Geometry: final body of the model. Coordinates: model frame, mm. A direction names the side the tool comes from. Give positions to 0.01 mm unless a question says otherwise; leave off trailing zeros. Write each loop counter-clockwise with the first axis right and the second up, starting at its lowest first coordinate (ties: lowest second). Pieces come first, ordered by that corner, then holes. Notation, with made-up numbers: (79.25, -10) -> (109.25, -10) arc R11 cw to (109.25, 3) -> close; hole circle Ø6 at (35, 68.25). An arc over 180 degrees is marked (long way). Use CSV: the item, a comma, the result in double quotes. Start each with the question number.
1) Material intervals for line 1 (Y direction, x = 249, z = 56); line 2 (Y direction, x = 108, z = 0), sorted ascending. Write a range as [from, to].
2) Contact query for flat-ended pins moving along their axis: P1, Ø6, axis at x = 129.5, y = -0.5, coming from the +Z side; P2, Ø1, axis at x = 158, y = 28, coming from the +Z side; P3, Ø24.5, axis at y = 97.86, z = -56.5, coming from the -X side. Output: stop coordinate, or through.
3) Section A-A (z = 99.5). Output: boundary loops of the cut face in (x, y), plus the area to 3 significant figures.
4) Draft query along X for faces 4 (the face through (13.846, 15.703, 37.874)), 5 (the face through (0, -10.6, 29.4)), 6 (the face through (1.479, 39.923, 20.765)). Return one class per face: pulls with the +X half, pulls with the -X half, needs draft (parallel to the pull), parting line crosses it, or undercut.
5) Section D-D (x = 57). Output: boundary loops of the cut face in (y, z), plus the area to 3 significant figures.
6) Section B-B (z = -113). Output: boundary loops of the cut face in (x, y), plus the area to 3 significant figures.
7) Set-up query: faces 1 (the face through (145.063, -15.77, 50.076)), 2 (the face through (106.482, -19.674, 62.475)), 3 (the face through (251.818, 59.354, -106.922)). Return all of +Z, -Z, +X, -X, +Y, -Y with unobstructed straight access to the full face (end or side cutting, diameter ignored); none if empty.
```python
from build123d import *

# Parameters (mm, degrees)
SKETCH_3_R           = 9.5
CUT_EXTRUDE_1_DEPTH  = 321.526909947
SKETCH_4_R           = 9.5
CUT_EXTRUDE_2_DEPTH  = 321.526909947
SKETCH_5_R           = 9.5
CUT_EXTRUDE_3_DEPTH  = 321.526909947
SKETCH_6_R           = 9.5
CUT_EXTRUDE_4_DEPTH  = 321.526909947
SKETCH_7_R           = 9.5
CUT_EXTRUDE_5_DEPTH  = 321.526909947
SKETCH_8_R           = 9.5
CUT_EXTRUDE_6_DEPTH  = 321.526909947
SKETCH_9_R           = 9.5
CUT_EXTRUDE_7_DEPTH  = 321.526909947
SKETCH_10_R          = 9.5
CUT_EXTRUDE_8_DEPTH  = 321.526909947
SKETCH_11_R          = 9.5
CUT_EXTRUDE_9_DEPTH  = 321.526909947
SKETCH_12_R          = 9.5
CUT_EXTRUDE_10_DEPTH = 321.526909947
SKETCH_13_R          = 9.5
CUT_EXTRUDE_11_DEPTH = 321.526909947
SKETCH_14_R          = 9.5
CUT_EXTRUDE_12_DEPTH = 321.526909947


with BuildPart() as part:
    # Эскиз1 → Повернуть1 (revolve)
    with BuildSketch(Plane.XY, mode=Mode.PRIVATE) as revolve_1_sk:
        Polygon((0, 0), (265, 0), (265, 127.5), (239, 127.5), (239, 100), (239, 95), (220, 95), (220, 94), (200, 94), (144, 65.5), (70, 65.5), (25, 41), (3, 41), (3, 45), (0, 45), align=None)
    revolve(revolve_1_sk.sketch.rotate(Axis((0, 0, 0), (1, 0, 0)), 90), axis=Axis((0, 0, 0), (1, 0, 0)))

    # Эскиз2 → Вырез-Повернуть1 (revolve, cut)
    with BuildSketch(Plane.XY, mode=Mode.PRIVATE) as cut_revolve_1_sk:
        with BuildLine():
            Line((0, 0), (239, 0))
            Line((239, 0), (239, 47))
            Line((239, 47), (210, 47))
            ThreePointArc((210, 47), (209, 47.16088641), (208, 47))
            Line((208, 47), (200, 55))
            Line((200, 55), (147.669872, 55))
            ThreePointArc((147.669872, 55), (146.273624348, 54.108499061), (146.669872, 52.5))
            Line((146.669872, 52.5), (143.5, 52.5))
            ThreePointArc((143.5, 52.5), (142.75, 52.602347572), (142, 52.5))
            Line((142, 52.5), (90, 52.5))
            ThreePointArc((90, 52.5), (79.13262933, 46.740617582), (70, 38.502577))
            Line((70, 38.502577), (42, 31))
            Line((42, 31), (0, 31))
            Line((0, 31), (0, 0))
        make_face()
    revolve(cut_revolve_1_sk.sketch.rotate(Axis((0, 0, 0), (1, 0, 0)), 90), axis=Axis((0, 0, 0), (1, 0, 0)), mode=Mode.SUBTRACT)

    # Эскиз3 → Вырез-Вытянуть1 (cut, through all)
    with BuildSketch(Plane(origin=(0, 0, 0), x_dir=(0, 0, -1), z_dir=(1, 0, 0))):
        with Locations((0, 113)):
            Circle(SKETCH_3_R)
    extrude(amount=CUT_EXTRUDE_1_DEPTH, mode=Mode.SUBTRACT)

    # Эскиз4 → Вырез-Вытянуть2 (cut, through all)
    with BuildSketch(Plane(origin=(0, 0, 0), x_dir=(0, 0, -1), z_dir=(1, 0, 0))):
        with Locations((-56.5, 97.860870628)):
            Circle(SKETCH_4_R)
    extrude(amount=CUT_EXTRUDE_2_DEPTH, mode=Mode.SUBTRACT)

    # Эскиз5 → Вырез-Вытянуть3 (cut, through all)
    with BuildSketch(Plane(origin=(0, 0, 0), x_dir=(0, 0, -1), z_dir=(1, 0, 0))):
        with Locations((-97.860870628, 56.5)):
            Circle(SKETCH_5_R)
    extrude(amount=CUT_EXTRUDE_3_DEPTH, mode=Mode.SUBTRACT)

    # Эскиз6 → Вырез-Вытянуть4 (cut, through all)
    with BuildSketch(Plane(origin=(0, 0, 0), x_dir=(0, 0, -1), z_dir=(1, 0, 0))):
        with Locations((-113, 0)):
            Circle(SKETCH_6_R)
    extrude(amount=CUT_EXTRUDE_4_DEPTH, mode=Mode.SUBTRACT)

    # Эскиз7 → Вырез-Вытянуть5 (cut, through all)
    with BuildSketch(Plane(origin=(0, 0, 0), x_dir=(0, 0, -1), z_dir=(1, 0, 0))):
        with Locations((-97.860870628, -56.5)):
            Circle(SKETCH_7_R)
    extrude(amount=CUT_EXTRUDE_5_DEPTH, mode=Mode.SUBTRACT)

    # Эскиз8 → Вырез-Вытянуть6 (cut, through all)
    with BuildSketch(Plane(origin=(0, 0, 0), x_dir=(0, 0, -1), z_dir=(1, 0, 0))):
        with Locations((-56.5, -97.860870628)):
            Circle(SKETCH_8_R)
    extrude(amount=CUT_EXTRUDE_6_DEPTH, mode=Mode.SUBTRACT)

    # Эскиз9 → Вырез-Вытянуть7 (cut, through all)
    with BuildSketch(Plane(origin=(0, 0, 0), x_dir=(0, 0, -1), z_dir=(1, 0, 0))):
        with Locations((0, -113)):
            Circle(SKETCH_9_R)
    extrude(amount=CUT_EXTRUDE_7_DEPTH, mode=Mode.SUBTRACT)

    # Эскиз10 → Вырез-Вытянуть8 (cut, through all)
    with BuildSketch(Plane(origin=(0, 0, 0), x_dir=(0, 0, -1), z_dir=(1, 0, 0))):
        with Locations((56.5, -97.860870628)):
            Circle(SKETCH_10_R)
    extrude(amount=CUT_EXTRUDE_8_DEPTH, mode=Mode.SUBTRACT)

    # Эскиз11 → Вырез-Вытянуть9 (cut, through all)
    with BuildSketch(Plane(origin=(0, 0, 0), x_dir=(0, 0, -1), z_dir=(1, 0, 0))):
        with Locations((97.860870628, -56.5)):
            Circle(SKETCH_11_R)
    extrude(amount=CUT_EXTRUDE_9_DEPTH, mode=Mode.SUBTRACT)

    # Эскиз12 → Вырез-Вытянуть10 (cut, through all)
    with BuildSketch(Plane(origin=(0, 0, 0), x_dir=(0, 0, -1), z_dir=(1, 0, 0))):
        with Locations((113, 0)):
            Circle(SKETCH_12_R)
    extrude(amount=CUT_EXTRUDE_10_DEPTH, mode=Mode.SUBTRACT)

    # Эскиз13 → Вырез-Вытянуть11 (cut, through all)
    with BuildSketch(Plane(origin=(0, 0, 0), x_dir=(0, 0, -1), z_dir=(1, 0, 0))):
        with Locations((97.860870628, 56.5)):
            Circle(SKETCH_13_R)
    extrude(amount=CUT_EXTRUDE_11_DEPTH, mode=Mode.SUBTRACT)

    # Эскиз14 → Вырез-Вытянуть12 (cut, through all)
    with BuildSketch(Plane(origin=(0, 0, 0), x_dir=(0, 0, -1), z_dir=(1, 0, 0))):
        with Locations((56.5, 97.860870628)):
            Circle(SKETCH_14_R)
    extrude(amount=CUT_EXTRUDE_12_DEPTH, mode=Mode.SUBTRACT)


solid = part.part
```
Answers follow:
1,line 1,"y = [-114.54, -107.35], [-88.37, 88.37], [107.35, 114.54]"
1,line 2,"y = [-65.5, -52.5], [52.5, 65.5]"
2,P1,"stops at z = 65.5"
2,P2,"stops at z = 67.36"
2,P3,"stops at x = 239"
3,outline,"(239, -79.72) -> (265, -79.72) -> (265, -65.86) -> (239, -65.86) -> close; (239, -47.14) -> (265, -47.14) -> (265, 47.14) -> (239, 47.14) -> close; (239, 65.86) -> (265, 65.86) -> (265, 79.72) -> (239, 79.72) -> close"
3,area,"3,170 mm^2"
4,face 4,"undercut"
4,face 5,"pulls with the -X half"
4,face 6,"needs draft"
5,outline,"circle Ø116.84 at (0, 0); hole circle Ø70.04 at (0, 0)"
5,area,"6,870 mm^2"
6,outline,"(239, -59.05) -> (265, -59.05) -> (265, -9.5) -> (239, -9.5) -> close; (239, 9.5) -> (265, 9.5) -> (265, 59.05) -> (239, 59.05) -> close"
6,area,"2,580 mm^2"
7,face 1,"none"
7,face 2,"-X"
7,face 3,"+X, -X"
